The model under review builds one solid part; all positions refer to its coordinate system, in mm. Round coordinates to 2 decimals unless told otherwise and drop trailing zeros. Answer as a JSON object with one key per item and string values. Group by question number.
1) To check wall thickness, follow probe 1 along Y at (x, z) = (420, 1.85); probe 2 along Y at (x, z) = (310, 0.5); probe 3 along Y at (x, z) = (281, 5). State the ranges of each line that lie inside material, in increasing order. Write a range as [from, to].
2) We need section A-A, the plane z = 4.25. Count the separate pieces of the cut face and the enclosed holes in it, then the cut area to 3 significant figures.
3) Insertion check: pin 1 Ø1 at (x, y) = (50, -432.5) entering from -Z; pin 2 Ø5 at (x, y) = (189.9, -189.9) entering from -Z. Each pin has a flat end and moves straight along its axis. Give the tip position at first contact, or say it passes through.
4) Mouldability with a two-part tool opening along X and no side actions: class faces 1 (the cylindrical face through (414.03, -410.64, 2.96)), 2 (the flat face through (247, -302, 6)) as pulls with the +X half, pulls with the -X half, needs draft (parallel to the pull), parting line crosses it, or undercut.
from build123d import *

# Parameters (mm, degrees)
SKETCH_1_W             = 500
SKETCH_1_H             = 500
EXTRUDE_1_DEPTH        = 6
SKETCH_2_W             = 90
SKETCH_2_H             = 90
CUT_EXTRUDE_565_DEPTH  = 7
CUT_EXTRUDE_1336_DEPTH = 7
SKETCH_4_R             = 4.5
SKETCH_4_R_2           = 2.6
CUT_EXTRUDE_2097_DEPTH = 7
CUT_EXTRUDE_3578_DEPTH = 7
SKETCH_7_R             = 4.05
SKETCH_7_R_2           = 2.6
CUT_EXTRUDE_4274_DEPTH = 7
SKETCH_8_R             = 2.6
CUT_EXTRUDE_4782_DEPTH = 7
SKETCH_5_R             = 11.1
SKETCH_5_R_2           = 1.6
SKETCH_5_R_3           = 1.55
CUT_EXTRUDE_4824_DEPTH = 7
SKETCH_9_R             = 2.5
CUT_EXTRUDE_4987_DEPTH = 7
SKETCH_10_R            = 1.6
MARK_DEPTH             = 7
SKETCH_11_W            = 2
SKETCH_11_H            = 3
CUT_EXTRUDE_5444_DEPTH = 7
SKETCH_12_R            = 4
CUT_EXTRUDE_5629_DEPTH = 7
SKETCH_13_R            = 2.1
CUT_EXTRUDE_3_DEPTH    = 7
SKETCH_14_R            = 5
CUT_EXTRUDE_4_DEPTH    = 7


with BuildPart() as part:
    # 草图1 → 凸台-拉伸1 (new body)
    with BuildSketch(Plane.XY):
        with Locations((250, -250)):
            Rectangle(SKETCH_1_W, SKETCH_1_H)
    extrude(amount=EXTRUDE_1_DEPTH)

    # 草图2 → Cut-Extrude 565 (cut, through all)
    with BuildSketch(Plane.XY.offset(6)):
        with Locations((250, -250)):
            Rectangle(SKETCH_2_W, SKETCH_2_H)
    extrude(amount=-CUT_EXTRUDE_565_DEPTH, mode=Mode.SUBTRACT)

    # 草图3 → Cut-Extrude 1336 (cut, through all)
    with BuildSketch(Plane.XY.offset(6)):
        with BuildLine():
            Line((248.4, -137), (248.4, -127))
            ThreePointArc((248.4, -127), (250, -125.4), (251.6, -127))
            Line((251.6, -127), (251.6, -137))
            ThreePointArc((251.6, -137), (250, -138.6), (248.4, -137))
        make_face()
        with BuildLine():
            Line((248.4, -197), (248.4, -187))
            ThreePointArc((248.4, -187), (250, -185.4), (251.6, -187))
            Line((251.6, -187), (251.6, -197))
            ThreePointArc((251.6, -197), (250, -198.6), (248.4, -197))
        make_face()
        with BuildLine():
            Line((248.4, -303), (248.4, -313))
            ThreePointArc((248.4, -313), (250, -314.6), (251.6, -313))
            Line((251.6, -313), (251.6, -303))
            ThreePointArc((251.6, -303), (250, -301.4), (248.4, -303))
        make_face()
        with BuildLine():
            Line((248.4, -363), (248.4, -373))
            ThreePointArc((248.4, -373), (250, -374.6), (251.6, -373))
            Line((251.6, -373), (251.6, -363))
            ThreePointArc((251.6, -363), (250, -361.4), (248.4, -363))
        make_face()
        with BuildLine():
            Line((187, -248.4), (197, -248.4))
            ThreePointArc((197, -248.4), (198.6, -250), (197, -251.6))
            Line((197, -251.6), (187, -251.6))
            ThreePointArc((187, -251.6), (185.4, -250), (187, -248.4))
        make_face()
        with BuildLine():
            Line((137, -251.6), (127, -251.6))
            ThreePointArc((127, -251.6), (125.4, -250), (127, -248.4))
            Line((127, -248.4), (137, -248.4))
            ThreePointArc((137, -248.4), (138.6, -250), (137, -251.6))
        make_face()
        with BuildLine():
            Line((313, -248.4), (303, -248.4))
            ThreePointArc((303, -248.4), (301.4, -250), (303, -251.6))
            Line((303, -251.6), (313, -251.6))
            ThreePointArc((313, -251.6), (314.6, -250), (313, -248.4))
        make_face()
        with BuildLine():
            Line((363, -251.6), (373, -251.6))
            ThreePointArc((373, -251.6), (374.6, -250), (373, -248.4))
            Line((373, -248.4), (363, -248.4))
            ThreePointArc((363, -248.4), (361.4, -250), (363, -251.6))
        make_face()
    extrude(amount=-CUT_EXTRUDE_1336_DEPTH, mode=Mode.SUBTRACT)

    # 草图4 → Cut-Extrude 2097 (cut, through all)
    with BuildSketch(Plane.XY.offset(6)):
        with Locations((420, -250)):
            Circle(SKETCH_4_R)
        with Locations((420, -268)):
            Circle(SKETCH_4_R_2)
        with Locations((420, -232)):
            Circle(SKETCH_4_R_2)
        with Locations((250, -420)):
            Circle(SKETCH_4_R)
        with Locations((232, -420)):
            Circle(SKETCH_4_R_2)
        with Locations((268, -420)):
            Circle(SKETCH_4_R_2)
        with Locations((80, -250)):
            Circle(SKETCH_4_R)
        with Locations((80, -232)):
            Circle(SKETCH_4_R_2)
        with Locations((80, -268)):
            Circle(SKETCH_4_R_2)
        with Locations((250, -80)):
            Circle(SKETCH_4_R)
        with Locations((268, -80)):
            Circle(SKETCH_4_R_2)
        with Locations((232, -80)):
            Circle(SKETCH_4_R_2)
    extrude(amount=-CUT_EXTRUDE_2097_DEPTH, mode=Mode.SUBTRACT)

    # 草图6 → Cut-Extrude 3578 (cut, through all)
    with BuildSketch(Plane(origin=(0, 0, 0), x_dir=(-1, 0, 0), z_dir=(0, 0, -1))):
        with BuildLine():
            Line((-174.818772789, -342.621985721), (-167.739030626, -349.684368528))
            ThreePointArc((-167.739030626, -349.684368528), (-167.734517194, -353.36132102), (-171.411469686, -353.365834453))
            Line((-171.411469686, -353.365834453), (-178.491211848, -346.303451645))
            ThreePointArc((-178.491211848, -346.303451645), (-178.495725281, -342.626499153), (-174.818772789, -342.621985721))
        make_face()
        with BuildLine():
            Line((-89.861866841, -427.370579408), (-82.782124679, -434.432962215))
            ThreePointArc((-82.782124679, -434.432962215), (-82.777611247, -438.109914707), (-86.454563739, -438.114428139))
            Line((-86.454563739, -438.114428139), (-93.534305901, -431.052045332))
            ThreePointArc((-93.534305901, -431.052045332), (-93.538819333, -427.37509284), (-89.861866841, -427.370579408))
        make_face()
        with BuildLine():
            Line((-72.347157479, -409.812818845), (-65.267415317, -416.875201653))
            ThreePointArc((-65.267415317, -416.875201653), (-61.590462825, -416.87068822), (-61.594976257, -413.193735728))
            Line((-61.594976257, -413.193735728), (-68.67471842, -406.131352921))
            ThreePointArc((-68.67471842, -406.131352921), (-72.351670912, -406.135866353), (-72.347157479, -409.812818845))
        make_face()
        with BuildLine():
            Line((-157.304063427, -325.064225159), (-150.224321264, -332.126607966))
            ThreePointArc((-150.224321264, -332.126607966), (-146.547368772, -332.122094534), (-146.551882205, -328.445142041))
            Line((-146.551882205, -328.445142041), (-153.631624367, -321.382759234))
            ThreePointArc((-153.631624367, -321.382759234), (-157.308576859, -321.387272667), (-157.304063427, -325.064225159))
        make_face()
        with BuildLine():
            Line((-132.385770641, -385.046305421), (-125.314702829, -392.117373233))
            ThreePointArc((-125.314702829, -392.117373233), (-125.314702829, -395.794328495), (-128.991658091, -395.794328495))
            Line((-128.991658091, -395.794328495), (-136.062725903, -388.723260683))
            ThreePointArc((-136.062725903, -388.723260683), (-136.062725903, -385.046305421), (-132.385770641, -385.046305421))
        make_face()
        with BuildLine():
            Line((-114.775699328, -367.392948508), (-107.687293483, -374.446635669))
            ThreePointArc((-107.687293483, -374.446635669), (-104.010349301, -374.437608811), (-104.019376159, -370.76066463))
            Line((-104.019376159, -370.76066463), (-111.107782004, -363.706977468))
            ThreePointArc((-111.107782004, -363.706977468), (-114.784726186, -363.716004326), (-114.775699328, -367.392948508))
        make_face()
    extrude(amount=-CUT_EXTRUDE_3578_DEPTH, mode=Mode.SUBTRACT)

    # 草图7 → Cut-Extrude 4274 (cut, through all)
    with BuildSketch(Plane(origin=(0, 0, 0), x_dir=(-1, 0, 0), z_dir=(0, 0, -1))):
        with Locations((-310.104076401, -310.104076401)):
            Circle(SKETCH_7_R)
        with Locations((-298.790367902, -321.4177849)):
            Circle(SKETCH_7_R_2)
        with Locations((-178.5822151, -201.209632098)):
            Circle(SKETCH_7_R_2)
        with Locations((-189.895923599, -189.895923599)):
            Circle(SKETCH_7_R)
        with Locations((-201.209632098, -178.5822151)):
            Circle(SKETCH_7_R_2)
        with Locations((-321.4177849, -298.790367902)):
            Circle(SKETCH_7_R_2)
    extrude(amount=-CUT_EXTRUDE_4274_DEPTH, mode=Mode.SUBTRACT)

    # 草图8 → Cut-Extrude 4782 (cut, through all)
    with BuildSketch(Plane(origin=(0, 0, 0), x_dir=(-1, 0, 0), z_dir=(0, 0, -1))):
        with Locations((-450, -10)):
            Circle(SKETCH_8_R)
        with Locations((-320, -10)):
            Circle(SKETCH_8_R)
        with Locations((-490, -50)):
            Circle(SKETCH_8_R)
        with Locations((-180, -10)):
            Circle(SKETCH_8_R)
        with Locations((-50, -10)):
            Circle(SKETCH_8_R)
        with Locations((-10, -180)):
            Circle(SKETCH_8_R)
        with Locations((-10, -50)):
            Circle(SKETCH_8_R)
        with Locations((-490, -450)):
            Circle(SKETCH_8_R)
        with Locations((-10, -320)):
            Circle(SKETCH_8_R)
        with Locations((-10, -450)):
            Circle(SKETCH_8_R)
        with Locations((-50, -490)):
            Circle(SKETCH_8_R)
        with Locations((-180, -490)):
            Circle(SKETCH_8_R)
        with Locations((-320, -490)):
            Circle(SKETCH_8_R)
        with Locations((-450, -490)):
            Circle(SKETCH_8_R)
    extrude(amount=-CUT_EXTRUDE_4782_DEPTH, mode=Mode.SUBTRACT)

    # 草图5 → Cut-Extrude 4824 (cut, through all)
    with BuildSketch(Plane(origin=(0, 0, 0), x_dir=(-1, 0, 0), z_dir=(0, 0, -1))):
        with Locations((-420, -420)):
            Circle(SKETCH_5_R)
        with Locations((-435.5, -404.5)):
            Circle(SKETCH_5_R_2)
        with Locations((-435.5, -435.5)):
            Circle(SKETCH_5_R_3)
        with Locations((-404.5, -435.5)):
            Circle(SKETCH_5_R_3)
        with Locations((-404.5, -404.5)):
            Circle(SKETCH_5_R_3)
    extrude(amount=-CUT_EXTRUDE_4824_DEPTH, mode=Mode.SUBTRACT)

    # 草图9 → Cut-Extrude 4987 (cut, through all)
    with BuildSketch(Plane(origin=(0, 0, 0), x_dir=(-1, 0, 0), z_dir=(0, 0, -1))):
        with Locations((-250, -115)):
            Circle(SKETCH_9_R)
        with Locations((-115, -250)):
            Circle(SKETCH_9_R)
        with Locations((-250, -385)):
            Circle(SKETCH_9_R)
        with Locations((-385, -250)):
            Circle(SKETCH_9_R)
    extrude(amount=-CUT_EXTRUDE_4987_DEPTH, mode=Mode.SUBTRACT)

    # 草图10 → mark (cut, through all)
    with BuildSketch(Plane(origin=(0, 0, 0), x_dir=(-1, 0, 0), z_dir=(0, 0, -1))):
        with Locations((-495, -295)):
            Circle(SKETCH_10_R)
        with Locations((-455, -295)):
            Circle(SKETCH_10_R)
        with Locations((-455, -205)):
            Circle(SKETCH_10_R)
        with Locations((-495, -205)):
            Circle(SKETCH_10_R)
    extrude(amount=-MARK_DEPTH, mode=Mode.SUBTRACT)

    # 草图11 → Cut-Extrude 5444 (cut, through all)
    with BuildSketch(Plane(origin=(0, 0, 0), x_dir=(-1, 0, 0), z_dir=(0, 0, -1))):
        with BuildLine():
            Line((-120, -287), (-110, -287))
            ThreePointArc((-110, -287), (-108.4, -288.6), (-110, -290.2))
            Line((-110, -290.2), (-120, -290.2))
            ThreePointArc((-120, -290.2), (-121.6, -288.6), (-120, -287))
        make_face()
        with Locations((-115, -271.6)):
            Rectangle(SKETCH_11_W, SKETCH_11_H)
    extrude(amount=-CUT_EXTRUDE_5444_DEPTH, mode=Mode.SUBTRACT)

    # 草图12 → Cut-Extrude 5629 (cut, through all)
    with BuildSketch(Plane(origin=(0, 0, 0), x_dir=(-1, 0, 0), z_dir=(0, 0, -1))):
        with Locations((-281.6, -140)):
            Circle(SKETCH_12_R)
        with Locations((-360, -281.6)):
            Circle(SKETCH_12_R)
        with Locations((-218.4, -360)):
            Circle(SKETCH_12_R)
        with Locations((-140, -218.4)):
            Circle(SKETCH_12_R)
    extrude(amount=-CUT_EXTRUDE_5629_DEPTH, mode=Mode.SUBTRACT)

    # 草图13 → 切除-拉伸3 (cut, through all)
    with BuildSketch(Plane(origin=(0, 0, 0), x_dir=(-1, 0, 0), z_dir=(0, 0, -1))):
        with Locations((-420, -360.485391833)):
            Circle(SKETCH_13_R)
        with Locations((-446.966991411, -53.033008589)):
            Circle(SKETCH_13_R)
        with Locations((-53.033008589, -53.033008589)):
            Circle(SKETCH_13_R)
        with Locations((-190.461090909, -309.538909091)):
            Circle(SKETCH_13_R)
        with Locations((-100.513688505, -143.317115932)):
            Circle(SKETCH_13_R)
        with Locations((-458.248464918, -140)):
            Circle(SKETCH_13_R)
        with Locations((-364.283495706, -96.516504294)):
            Circle(SKETCH_13_R)
        with Locations((-409.215443709, -152.251775839)):
            Circle(SKETCH_13_R)
    extrude(amount=-CUT_EXTRUDE_3_DEPTH, mode=Mode.SUBTRACT)

    # 草图14 → 切除-拉伸4 (cut, through all)
    with BuildSketch(Plane(origin=(0, 0, 0), x_dir=(-1, 0, 0), z_dir=(0, 0, -1))):
        with Locations((-218.4, -140)):
            Circle(SKETCH_14_R)
    extrude(amount=-CUT_EXTRUDE_4_DEPTH, mode=Mode.SUBTRACT)


solid = part.part
Here are the results:
{
 "1": {"probe 1": "y = [-500, -431.1], [-408.9, -362.59], [-358.39, -270.6], [-265.4, -254.5], [-245.5, -234.6], [-229.4, 0]", "probe 2": "y = [-500, -314.15], [-306.06, -251.6], [-248.4, 0]", "probe 3": "y = [-500, -295], [-205, -143.95], [-136.05, 0]"},
 "2": {"separate pieces": "1", "enclosed holes": "75", "area": "239,000 mm^2"},
 "3": {"pin 1": "stops at z = 0", "pin 2": "passes through"},
 "4": {"face 1": "undercut", "face 2": "needs draft"}
}
